Autodesk Inventor part; units mm, degrees
ref_plane "YZ Plane" through (0, 0, 0) normal (1, 0, 0) x (0, 1, 0)
ref_plane "XZ Plane" through (0, 0, 0) normal (0, 1, 0) x (-1, 0, 0)
ref_plane "XY Plane" through (0, 0, 0) normal (0, 0, 1) x (1, 0, 0)
sketch "Sketch5" plane through (0, 0, 0) normal (1, 0, 0) x (0, 1, 0)
  circle A0 centre (0, 0) radius 5.5
  dimension "d11" = 11
extrude "Extrusion5" add sketch "Sketch5" along normal blind 4
sketch "Sketch7" plane through (4, 0, 0) normal (1, 0, 0) x (0, 0, -1)
  circle A0 centre (0, 0) radius 5.5
hole "Hole1" at (4, 0, 0) direction (-1, 0, 0) diameter 3.121 end through all counterbore diameter 5.3 counterbore depth 2.4
sketch "Sketch10" plane through (4, 0, 0) normal (1, 0, 0) x (0, 0, -1)
  line L0 (-2.7575, 3.0003) -> (2.7575, 3.0003)
  line L1 (2.7575, -3.0003) -> (-2.7575, -3.0003)
  line L2 (-2.7575, 3.0003) -> (2.7575, -3.0003) construction
  line L3 (2.7575, 3.0003) -> (-2.7575, -3.0003) construction
  arc A0 (2.7575, 3.0003) -> (-2.7575, 3.0003) centre (0, 0) ccw
  arc A1 (-2.7575, -3.0003) -> (2.7575, -3.0003) centre (0, 0) ccw
extrude "Extrusion8" add sketch "Sketch10" along normal blind 5
sketch "Sketch11" plane through (4, 0, 0) normal (1, 0, 0) x (0, 0, -1)
  circle A0 centre (0, 0) radius 1.5605
  circle A1 centre (0, 0) radius 4.075
  circle A2 centre (0, 0) radius 5.5
sketch "Sketch12" plane through (0, 0, 0) normal (-1, 0, 0) x (0, 0, 1)
  circle A0 centre (0, 0) radius 2.975
  circle A1 centre (0, 0) radius 5.5
  dimension "d35" = 5.95
extrude "Extrusion10" add sketch "Sketch12" along normal blind 3.5
extrude "Extrusion11" add sketch "Sketch11" along normal blind 5 contours A2
fillet "Fillet4" radius 1 1 edges at (-3.5, 0, -5.5)
fillet "Fillet4" radius 0.5 1 edges at (9, 0, 5.5)
properties part number "servo_adapter"
Here's how the part is built. I have some questions about the finished solid (model axes, mm). A direction names the side the tool comes from. Coordinates: 2 decimals unless noted, no trailing zeros. Order: outer loops, then holes, each group sorted by start corner. A loop starts at its lowest first (then second) coordinate and runs counter-clockwise, first axis right, second up. Notation, with made-up numbers: (80, 71) - (129, 71) arc R24 ccw to (129, 109) - close; hole circle Ø2 at (6, 29). An arc over 180 degrees is marked (long way). One line per question, with ' | ' between items. Start each with the question number.
1. Please list where these lines run through material, in increasing order: line 1 along Z through (x, y) = (3.3, 0); line 2 along Y through (x, z) = (0.6, 0); line 3 along Y through (x, z) = (-2, 0) (3 decimals). Write a range as [from, to].
2. Which directions (+Z, -Z, +X, -X, +Y, -Y) give clear straight access to the entire face, cutting with the end or side of a thin tool? Please do faces 3 (the flat face through (4, -2, -2)), 4 (the flat face through (-3.5, -3, 1)), 5 (the cylindrical face through (-1.7, -2, -2.2)).
3. If we section it at D-D (x = 1): Write out the boundary of the cut face in (y, z), and give its area (3 significant figures).
4. I'm going to push flat-ended pins straight in: pin 1 Ø3 at (y, z) = (1, -0.5) entering from -X; pin 2 Ø1 at (x, z) = (3, -3) entering from +Y; pin 3 Ø1.6 at (y, z) = (-0.5, 1) entering from +X. Where does each tip first touch, or does it pass through?
5. If we mould it in two halves opening along Z, with no side actions, what happens to faces 1 (the flat face through (9, -3.3, 0.1)), 2 (the flat face through (6, 3, 0))? For each: released by +Z, released by -Z, zero draft, split by the parting line, or undercut.
6. If we section it at C-C (x = 2.25): Write out the boundary of the cut face in (y, z).
Model answer:
1) line 1: z = [-5.5, -2.65], [2.65, 5.5] | line 2: y = [-5.5, -1.56], [1.56, 5.5] | line 3: y = [-5.5, -2.975], [2.975, 5.5]
2) face 3: +X | face 4: +Z, -Z, -X, +Y, -Y | face 5: -X
3) outline: circle Ø11 at (0, 0); hole circle Ø3.12 at (0, 0) | area: 87.4 mm²
4) pin 1: stops at x = 0 | pin 2: stops at y = 4.9 | pin 3: stops at x = 1.6
5) face 1: zero draft | face 2: undercut
6) outline: circle Ø11 at (0, 0); hole circle Ø5.3 at (0, 0)
